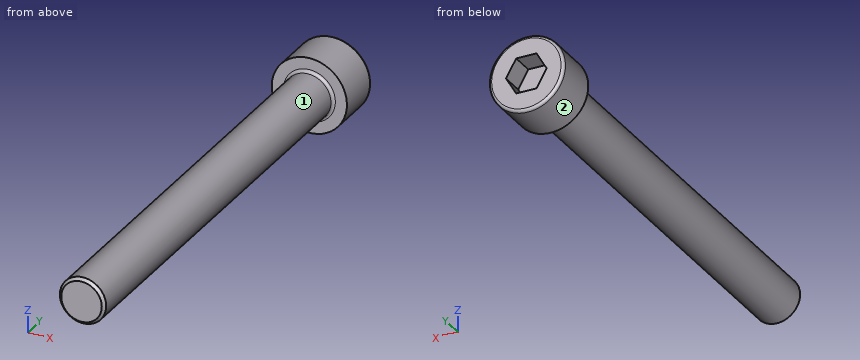
from build123d import *

# Parameters (mm, degrees)
SKETCH_1_R          = 6.5
EXTRUDE_1_DEPTH     = 8
CUT_EXTRUDE_1_DEPTH = 4
FILLET_1_R          = 0.5
SKETCH_3_R          = 4
EXTRUDE_2_DEPTH     = 75
FILLET_2_R          = 0.5
CHAMFER_1_SIZE      = 0.5


with BuildPart() as part:
    # ｽｹｯﾁ1 → ﾎﾞｽ - 押し出し1 (new body)
    with BuildSketch(Plane(origin=(0, 0, 0), x_dir=(1, 0, 0), z_dir=(0, 1, 0))):
        with Locations(Location((0, 0, 0), (0, 0, 270))):
            Circle(SKETCH_1_R)
    extrude(amount=EXTRUDE_1_DEPTH)

    # ｽｹｯﾁ2 → ｶｯﾄ - 押し出し1 (cut)
    with BuildSketch(Plane(origin=(0, 8, 0), x_dir=(1, 0, 0), z_dir=(0, 1, 0))):
        Polygon((3.516063139, 0), (1.75803157, 3.045), (-1.75803157, 3.045), (-3.516063139, 0), (-1.75803157, -3.045), (1.75803157, -3.045), align=None)
    extrude(amount=-CUT_EXTRUDE_1_DEPTH, mode=Mode.SUBTRACT)

    # ﾌｨﾚｯﾄ1
    fillet_1_edges = [part.edges().sort_by_distance(p)[0] for p in [
        (0, 8, -6.5),
    ]]
    fillet(fillet_1_edges, radius=FILLET_1_R)

    # ｽｹｯﾁ3 → ﾎﾞｽ - 押し出し2 (add)
    with BuildSketch(Plane.XZ):
        with Locations(Location((0, 0, 0), (0, 0, 90))):
            Circle(SKETCH_3_R)
    extrude(amount=EXTRUDE_2_DEPTH)

    # ﾌｨﾚｯﾄ2
    fillet_2_edges = [part.edges().sort_by_distance(p)[0] for p in [
        (0, 0, -4),
    ]]
    fillet(fillet_2_edges, radius=FILLET_2_R)

    # 面取り1
    chamfer_1_edges = [part.edges().sort_by_distance(p)[0] for p in [
        (0, -75, -4),
    ]]
    chamfer(chamfer_1_edges, length=CHAMFER_1_SIZE)


solid = part.part
Here's how the part is built. I have some questions about the finished solid (model axes, mm). Face numbers are marked on the shaded views. A direction names the side the tool comes from. Coordinates: 2 decimals unless noted, no trailing zeros. Order: outer loops, then holes, each group sorted by start corner. A loop starts at its lowest first (then second) coordinate and runs counter-clockwise, first axis right, second up. Notation, with made-up numbers: M 55,-18 L 66,-18 A14 ccw 66,7 Z; hole C 31,18 d11. An arc over 180 degrees is marked long. Answer as CSV lines item,"result". Start each with the question number.
1. On a 3-axis mill with a long thin cutter (end or side, diameter ignored), from which of +Z, -Z, +X, -X, +Y, -Y can I reach the whole of each face in a straight line? I mean the marked faces 1 and 2. Say none if no direction works.
2. I need wall thicknesses on line 1 (Y direction, x = -5.5, z = -0.25); line 2 (Y direction, x = -2.5, z = -0.5); line 3 (X direction, y = 5, z = -5.75). Which ranges of each line are inside material? Lowest first, please. Write a range as [from, to].
3. I want a section at A-A, the plane x = 0. Write out the boundary of the cut face in (y, z) (3 decimals).
4. For pin 1 (1.5 mm diameter, centred on x = 3, z = 5, fed in from -Y); pin 2 (1 mm diameter, centred on x = 0.5, y = -66, fed in from +Z); pin 3 (3 mm diameter, centred on y = -39, z = 3, fed in from +X), each with a flat end and sliding along its axis, tell me the tip position at first contact or that it passes through.
5. I want a section at B-B, the plane y = -62. Write out the boundary of the cut face in (x, z), and give its area (3 significant figures).
Recorded:
1,face 1,"-Y"
1,face 2,"+Y, -Y"
2,line 1,"y = [0, 8]"
2,line 2,"y = [-75, 4]"
2,line 3,"x = [-3.03, 3.03]"
3,outline,"M -75,-3.5 L -74.5,-4 L -0.5,-4 A0.5 cw 0,-4.5 L 0,-6.5 L 7.5,-6.5 A0.5 ccw 8,-6 L 8,-3.045 L 4,-3.045 L 4,3.045 L 8,3.045 L 8,6 A0.5 ccw 7.5,6.5 L 0,6.5 L 0,4.5 A0.5 cw -0.5,4 L -74.5,4 L -75,3.5 Z"
4,pin 1,"stops at y = 0"
4,pin 2,"stops at z = 4"
4,pin 3,"stops at x = 3.71"
5,outline,"C 0,0 d8"
5,area,"50.3 mm2"
